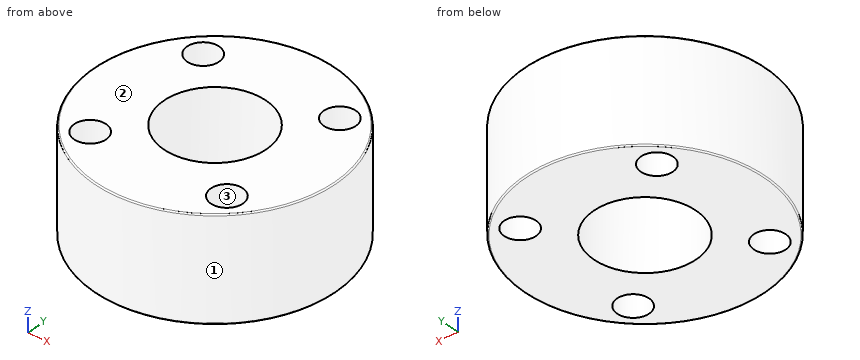
from build123d import *

# Parameters (mm, degrees)
SKETCH_1_R      = 9.43812854
SKETCH_1_R_2    = 4
SKETCH_1_R_3    = 1.25
EXTRUDE_1_DEPTH = 8
FILLET_1_R      = 0.1


with BuildPart() as part:
    # Эскиз1 → Бобышка-Вытянуть1 (new body)
    with BuildSketch(Plane.XY):
        Circle(SKETCH_1_R)
        Circle(SKETCH_1_R_2, mode=Mode.SUBTRACT)
        with Locations((-5.325171984, 5.281339162)):
            Circle(SKETCH_1_R_3, mode=Mode.SUBTRACT)
        with Locations((-5.281339162, -5.325171984)):
            Circle(SKETCH_1_R_3, mode=Mode.SUBTRACT)
        with Locations((5.325171984, -5.281339162)):
            Circle(SKETCH_1_R_3, mode=Mode.SUBTRACT)
        with Locations((5.281339162, 5.325171984)):
            Circle(SKETCH_1_R_3, mode=Mode.SUBTRACT)
    extrude(amount=EXTRUDE_1_DEPTH)

    # Скругление1
    fillet_1_edges = [part.edges().sort_by_distance(p)[0] for p in [
        (-9.43812854, 0, 0),
        (-9.43812854, 0, 8),
    ]]
    fillet(fillet_1_edges, radius=FILLET_1_R)


solid = part.part
Work out the finished part from the listing and answer in its coordinate system (mm). Face numbers are marked on the shaded views. Give positions to 0.01 mm unless a question says otherwise; leave off trailing zeros. Write each loop counter-clockwise with the first axis right and the second up, starting at its lowest first coordinate (ties: lowest second). Pieces come first, ordered by that corner, then holes.
Q1. The part is cut by section D-D on x = 6. State how many separate pieces and enclosed holes the cut face has, and give its area (3 significant figures).
Answer:
separate pieces: 3
enclosed holes: 0
area: 83.4 mm2
Q2. The part is cut by section A-A on y = 0. Give the vertices of the cut face in (x, z), and give its area (3 significant figures).
Answer:
outline: (-9.44, 0.1) arc R0.1 ccw to (-9.34, 0) - (-4, 0) - (-4, 8) - (-9.34, 8) arc R0.1 ccw to (-9.44, 7.9) - close; (4, 0) - (9.34, 0) arc R0.1 ccw to (9.44, 0.1) - (9.44, 7.9) arc R0.1 ccw to (9.34, 8) - (4, 8) - close
area: 87.0 mm2
Q3. For a pull along Y with two mould halves and no side action, classify the marked faces 1, 2 and 3 as released by +Y, released by -Y, zero draft, split by the parting line, or undercut.
Answer:
face 1: split by the parting line
face 2: zero draft
face 3: undercut
Q4. Straight lines are drawn through the part: L1, parallel to Y at x = 0, z = 4; L2, parallel to Y at x = 6, z = 3; L3, parallel to X at y = -6.25, z = 2.5. For each, find the intervals that lie inside material, in ascending order.
Answer:
L1: y = -9.44 to -4, 4 to 9.44
L2: y = -7.29 to -6.33, -4.23 to 4.3, 6.35 to 7.29
L3: x = -7.07 to -6.12, -4.44 to 4.54, 6.12 to 7.07
Q5. The part is cut by section C-C on z = 0.5. Give the vertices of the cut face in (x, y), and give its area (3 significant figures).
Answer:
outline: circle Ø18.88 at (0, 0); hole circle Ø2.5 at (-5.33, 5.28); hole circle Ø2.5 at (-5.28, -5.33); hole circle Ø8 at (0, 0); hole circle Ø2.5 at (5.28, 5.33); hole circle Ø2.5 at (5.33, -5.28)
area: 210 mm2
Q6. Given pin 1 (1.5 mm diameter, centred on y = -4, z = 7, fed in from +X); pin 2 (4 mm diameter, centred on y = 2.5, z = 1, fed in from +X); pin 3 (1 mm diameter, centred on y = 4.5, z = 6, fed in from +X); pin 4 (1.5 mm diameter, centred on x = 5.33, y = -5.28, fed in from -Z), each flat-ended and moving along its own axis, determine where each tip first touches the part or whether it passes through.
Answer:
pin 1: stops at x = 8.86
pin 2: stops at x = 9.42
pin 3: stops at x = 8.55
pin 4: passes through
